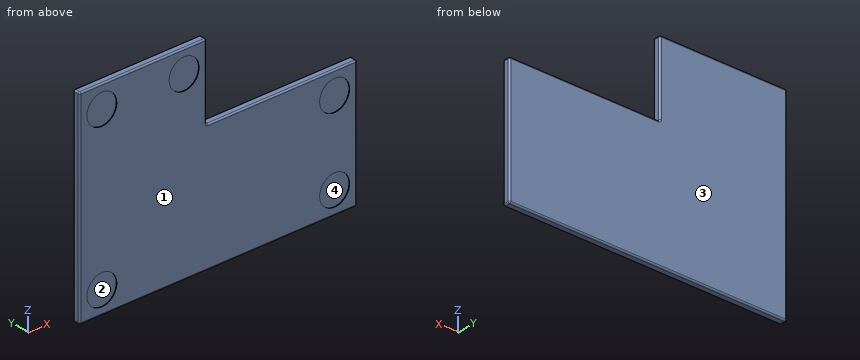
from build123d import *

# Parameters (mm, degrees)
F1_DEPTH = 25.4
F3_R     = 50.8
F4_DEPTH = 2.54
F5_R     = 5.08


with BuildPart() as f1:
    # F0 (on Front) → F1 (new body)
    with BuildSketch(Plane.XZ):
        Polygon((-471.4875, -342.9), (471.4875, -342.9), (471.4875, 88.9), (-39.6875, 88.9), (-39.6875, 342.9), (-471.4875, 342.9), align=None)
    extrude(amount=F1_DEPTH)

    # F3 (on face) → F4 (cut)
    with BuildSketch(Plane.XZ.offset(25.4)):
        with Locations((-395.2875, 266.7)):
            Circle(F3_R)
        with Locations((-115.8875, 266.7)):
            Circle(F3_R)
        with Locations((-395.2875, -266.7)):
            Circle(F3_R)
        with Locations((395.2875, -266.7)):
            Circle(F3_R)
        with Locations((395.2875, 12.7)):
            Circle(F3_R)
    extrude(amount=-F4_DEPTH, mode=Mode.SUBTRACT)

    # F5
    f5_edges = [f1.edges().sort_by_distance(p)[0] for p in [
        (-471.4875, -12.7, -342.9),
        (471.4875, -12.7, -342.9),
        (0, 0, -342.9),
        (0, -25.4, -342.9),
        (-471.4875, -12.7, 342.9),
        (-471.4875, 0, 0),
        (-471.4875, -25.4, 0),
        (471.4875, -12.7, 88.9),
        (471.4875, 0, -127),
        (471.4875, -25.4, -127),
        (-39.6875, -12.7, 88.9),
        (215.9, 0, 88.9),
        (215.9, -25.4, 88.9),
        (-39.6875, -12.7, 342.9),
        (-39.6875, 0, 215.9),
        (-39.6875, -25.4, 215.9),
        (-255.5875, 0, 342.9),
        (-255.5875, -25.4, 342.9),
    ]]
    fillet(f5_edges, radius=F5_R)


solid = f1.part
Part model, mm, in its own coordinate system. Face numbers are marked on the shaded views. A direction names the side the tool comes from. Give positions to 0.01 mm unless a question says otherwise; leave off trailing zeros. Write each loop counter-clockwise with the first axis right and the second up, starting at its lowest first coordinate (ties: lowest second). Pieces come first, ordered by that corner, then holes.
1) Probe L1, parallel to Z at x = 91, y = -8.5; L2, parallel to Z at x = -231.5, y = -21.25; L3, parallel to X at y = -4.5, z = 69.5. List the from-to ranges inside material, lowest first.
Resolved:
L1: z = -342.9 to 88.9
L2: z = -342.81 to 342.81
L3: x = -471.45 to 471.45
2) Cut at C-C on y = -16. Write the cut outline in (x, z).
Resolved:
outline: (-471.49, -337.82) arc R5.08 ccw to (-466.41, -342.9) - (466.41, -342.9) arc R5.08 ccw to (471.49, -337.82) - (471.49, 83.82) arc R5.08 ccw to (466.41, 88.9) - (-34.61, 88.9) arc R5.08 cw to (-39.69, 93.98) - (-39.69, 337.82) arc R5.08 ccw to (-44.77, 342.9) - (-466.41, 342.9) arc R5.08 ccw to (-471.49, 337.82) - close
3) Cut at A-A on z = 266.7. Write the cut outline in (x, y).
Resolved:
outline: (-471.49, -20.32) arc R5.08 ccw to (-466.41, -25.4) - (-446.09, -25.4) - (-446.09, -22.86) - (-344.49, -22.86) - (-344.49, -25.4) - (-166.69, -25.4) - (-166.69, -22.86) - (-65.09, -22.86) - (-65.09, -25.4) - (-44.77, -25.4) arc R5.08 ccw to (-39.69, -20.32) - (-39.69, -5.08) arc R5.08 ccw to (-44.77, 0) - (-466.41, 0) arc R5.08 ccw to (-471.49, -5.08) - close
4) Which spindle directions (+Z, -Z, +X, -X, +Y, -Y) get a long thin tool onto all of the face, cutting with end or side? Do the marked faces 3 and 4. Say none if no direction does.
Resolved:
face 3: +Z, -Z, +X, -X, +Y
face 4: -Y
5) Pin check, flat tips, straight feed: pin 1 (1 mm diameter, centred on x = -142.5, z = -267, fed in from +Y); pin 2 (1 mm diameter, centred on x = 230, y = -9.5, fed in from +Z); pin 3 (12 mm diameter, centred on y = -9, z = 156, fed in from +X). Stop position of each tip, or through.
Resolved:
pin 1: stops at y = 0
pin 2: stops at z = 88.9
pin 3: stops at x = -39.69
6) Cut at D-D on z = -266.7. Write the cut outline in (x, y), then the cut area to 3 significant figures.
Resolved:
outline: (-471.49, -20.32) arc R5.08 ccw to (-466.41, -25.4) - (-446.09, -25.4) - (-446.09, -22.86) - (-344.49, -22.86) - (-344.49, -25.4) - (344.49, -25.4) - (344.49, -22.86) - (446.09, -22.86) - (446.09, -25.4) - (466.41, -25.4) arc R5.08 ccw to (471.49, -20.32) - (471.49, -5.08) arc R5.08 ccw to (466.41, 0) - (-466.41, 0) arc R5.08 ccw to (-471.49, -5.08) - close
area: 23,400 mm2
7) Cut at B-B on x = 101. Write the cut outline in (y, z).
Resolved:
outline: (-25.4, -337.82) arc R5.08 ccw to (-20.32, -342.9) - (-5.08, -342.9) arc R5.08 ccw to (0, -337.82) - (0, 83.82) arc R5.08 ccw to (-5.08, 88.9) - (-20.32, 88.9) arc R5.08 ccw to (-25.4, 83.82) - close
8) Two-plate mould, pull along X, no slides. Class the marked faces 1 and 2: released by +X, released by -X, zero draft, split by the parting line, or undercut.
Resolved:
face 1: zero draft
face 2: undercut
